Design review of the part built by this model. Coordinates are the model's own, in mm. A direction names the side the tool comes from. Coordinates: 2 decimals unless noted, no trailing zeros. Loops run counter-clockwise (first coordinate to the right, second up) from the corner with the lowest first, then second, coordinate; pieces in that order, holes last.
Q1. Wall thickness on probe 1 along Y at (x, z) = (-2, -98.5); probe 2 along X at (y, z) = (19, -122); probe 3 along Y at (x, z) = (0.5, 67): over which ranges is each line inside the solid? List them lowest first.
Q2. Add section C-C on z = -67.5. Give the boundary of the cut face in (x, y), and give its area (3 significant figures).
Q3. Machinability: for faces 1 (the face through (-19.05, 28, -129)), 2 (the face through (0, 19, 114.3)), 3 (the face through (0, 12.7, -44)), 4 (the face through (0, 38.1, -17)), 5 (the face through (19.05, 28, -129)), which of the approach directions +Z, -Z, +X, -X, +Y, -Y give a long, thin tool a straight path to every point of the face, cutting with its end or side? Answer none if there is none.
Q4. Add section B-B on x = -11.5. Give the boundary of the cut face in (y, z), and give its area (3 significant figures).
Q5. For P1, Ø1, axis at y = 11.5, z = 24.5, coming from the +X side; P2, Ø1, axis at x = 10, y = 12.5, coming from the -Z side; P3, Ø12, axis at y = 10, z = -84, coming from the +X side; P4, Ø14, axis at x = -5, z = -75.5, coming from the -Y side, all flat-tipped, find the tip position at first contact; note any pin that passes through.
Q6. Add section A-A on y = 26. Give the boundary of the cut face in (x, z), and give its area (3 significant figures).
Q7. Add section D-D on y = 3. Give the boundary of the cut face in (x, z).
```python
from build123d import *

# Parameters (mm, degrees)
SKETCH1_W           = 38.1
SKETCH1_H           = 38.1
BOSS_EXTRUDE2_DEPTH = 50.8
SKETCH11_W          = 266.7
SKETCH11_H          = 12.7
CUT_EXTRUDE6_DEPTH  = 51.8


with BuildPart() as part:
    # Sketch1 → Boss-Extrude2 (new body)
    with BuildSketch(Plane(origin=(0, 0, 0), x_dir=(1, 0, 0), z_dir=(0, 1, 0))):
        Polygon((-19.05, 114.3), (-25.4, -114.3), (25.4, -114.3), (19.05, 114.3), align=None)
        with Locations((0, 133.35)):
            Rectangle(SKETCH1_W, SKETCH1_H)
    extrude(amount=BOSS_EXTRUDE2_DEPTH)

    # Sketch11 → Cut-Extrude6 (cut, through all)
    with BuildSketch(Plane(origin=(25.4, 0, 0), x_dir=(0, 0, -1), z_dir=(1, 0, 0))):
        Polygon((114.3, 12.7), (-29.077687403, 12.7), (-114.3, 0), (152.4, 0), (152.4, 12.7), align=None)
        with Locations((19.05, 44.45)):
            Rectangle(SKETCH11_W, SKETCH11_H)
        Polygon((152.4, 12.7), (152.4, 31.75), (114.3, 12.7), align=None)
    extrude(amount=-CUT_EXTRUDE6_DEPTH, mode=Mode.SUBTRACT)


solid = part.part
```
Entries:
1. probe 1: y = 12.7 to 38.1
1. probe 2: x = -19.05 to 19.05
1. probe 3: y = 7.05 to 38.1
2. outline: (-20.35, 12.7) - (20.35, 12.7) - (20.35, 38.1) - (-20.35, 38.1) - close
2. area: 1,030 mm2
3. face 1: -Z, -X, +Y, -Y
3. face 2: +Z, +X, -X, +Y, -Y
3. face 3: -Z, +X, -X, -Y
3. face 4: +Z, -Z, +X, -X, +Y
3. face 5: -Z, +X, +Y, -Y
4. outline: (0, 114.3) - (12.7, 29.08) - (12.7, -114.3) - (31.75, -152.4) - (38.1, -152.4) - (38.1, 114.3) - close
4. area: 6,950 mm2
5. P1: passes through
5. P2: stops at z = -114.9
5. P3: stops at x = 20.04
5. P4: stops at y = 12.7
6. outline: (-25.4, 114.3) - (-19.05, -114.3) - (-19.05, -140.9) - (19.05, -140.9) - (19.05, -114.3) - (25.4, 114.3) - close
6. area: 11,200 mm2
7. outline: (-25.4, 114.3) - (-24.84, 94.17) - (24.84, 94.17) - (25.4, 114.3) - close
